```python
from build123d import *

# Parameters (mm, degrees)
F1_DEPTH  = 2
F2_W      = 78
F2_H      = 1.5
F3_DEPTH  = 2
F4_W      = 20
F4_H      = 1.5
F5_DEPTH  = 7
F6_W      = 78
F6_H      = 1.5
F7_DEPTH  = 2
F8_W      = 78
F8_H      = 3
F9_DEPTH  = 3
F10_DEPTH = 2
F11_DEPTH = 2
F12_W     = 3
F12_H     = 11
F13_DEPTH = 5
F14_R     = 5


with BuildPart() as f1:
    # F0 (on Top) → F1 (new body)
    with BuildSketch(Plane.XY):
        with BuildLine():
            Line((7.8453938663, 18.7269745824), (-14.6546061337, 18.7269745824))
            add(Edge.make_bspline(
                [(-14.6546061337, 18.7269745824), (-14.6546061337, 12.4846497216), (-14.9176308165, 6.2423248608), (-15.345167051, 0)],
                knots=[0.5, 0.5, 0.5, 0.5, 0.6872697458, 0.6872697458, 0.6872697458, 0.6872697458], degree=3))
            Line((-15.345167051, 0), (8.5359547836, 0))
            add(Edge.make_bspline(
                [(7.8453938663, 18.7269745824), (7.8453938663, 12.4846497216), (8.1084185491, 6.2423248608), (8.5359547836, 0)],
                knots=[0.5, 0.5, 0.5, 0.5, 0.6872697458, 0.6872697458, 0.6872697458, 0.6872697458], degree=3))
        make_face()
        Polygon((11.5953938663, -31.2730254176), (-18.4046061337, -31.2730254176), (-42.4046061337, -31.2730254176), (-42.4046061337, -34.2730254176), (35.5953938663, -34.2730254176), (35.5953938663, -31.2730254176), align=None)
        with BuildLine():
            Line((8.5359547836, 0), (-15.345167051, 0))
            add(Edge.make_bspline(
                [(-15.345167051, 0), (-16.0591292274, -10.4243418059), (-17.2318676805, -20.8486836117), (-18.4046061337, -31.2730254176)],
                knots=[0.6872697458, 0.6872697458, 0.6872697458, 0.6872697458, 1, 1, 1, 1], degree=3))
            Line((-18.4046061337, -31.2730254176), (11.5953938663, -31.2730254176))
            add(Edge.make_bspline(
                [(8.5359547836, 0), (9.24991696, -10.4243418059), (10.4226554131, -20.8486836117), (11.5953938663, -31.2730254176)],
                knots=[0.6872697458, 0.6872697458, 0.6872697458, 0.6872697458, 1, 1, 1, 1], degree=3))
        make_face()
    extrude(amount=F1_DEPTH)

    # F2 (on face) → F3 (join)
    with BuildSketch(Plane.XY.offset(2)):
        with Locations((-3.4046061337, -33.5230254176)):
            Rectangle(F2_W, F2_H)
    extrude(amount=F3_DEPTH)

    # F4 (on face) → F5 (join)
    with BuildSketch(Plane.XY.offset(4)):
        with Locations((-32.4046061337, -33.5230254176)):
            Rectangle(F4_W, F4_H)
        with Locations((25.5953938663, -33.5230254176)):
            Rectangle(F4_W, F4_H)
    extrude(amount=F5_DEPTH)

    # F6 (on face) → F7 (join)
    with BuildSketch(Plane.XY.offset(11)):
        with Locations((-3.4046061337, -33.5230254176)):
            Rectangle(F6_W, F6_H)
    extrude(amount=F7_DEPTH)

    # F8 (on face) → F9 (join)
    with BuildSketch(Plane.XY.offset(13)):
        with Locations((-3.4046061337, -32.7730254176)):
            Rectangle(F8_W, F8_H)
    extrude(amount=F9_DEPTH)

    # F10 (add): a face of the model
    f10_faces = [f1.faces().sort_by_distance(p)[0] for p in [
        (-3.4046061337, -31.2730254176, 14.5),
    ]]
    extrude(f10_faces, amount=F10_DEPTH)

    # F11 (add): faces of the model
    f11_faces = [f1.faces().sort_by_distance(p)[0] for p in [
        (23.5953938663, -31.2730254176, 1),
        (-30.4046061337, -31.2730254176, 1),
    ]]
    extrude(f11_faces, amount=F11_DEPTH)

    # F12 (on face) → F13 (join)
    with BuildSketch(Plane(origin=(0, -32.7730254176, 0), x_dir=(-1, 0, 0), z_dir=(0, 1, 0))):
        with Locations((40.9046061337, 7.5)):
            Rectangle(F12_W, F12_H)
        with Locations((-34.0953938663, 7.5)):
            Rectangle(F12_W, F12_H)
    extrude(amount=F13_DEPTH)

    # F14
    f14_edges = [f1.edges().sort_by_distance(p)[0] for p in [
        (35.595394, -31.773025, 16),
        (35.595394, -31.773025, 0),
        (-42.404606, -31.773025, 0),
        (-42.404606, -31.773025, 16),
    ]]
    fillet(f14_edges, radius=F14_R)


solid = f1.part
```
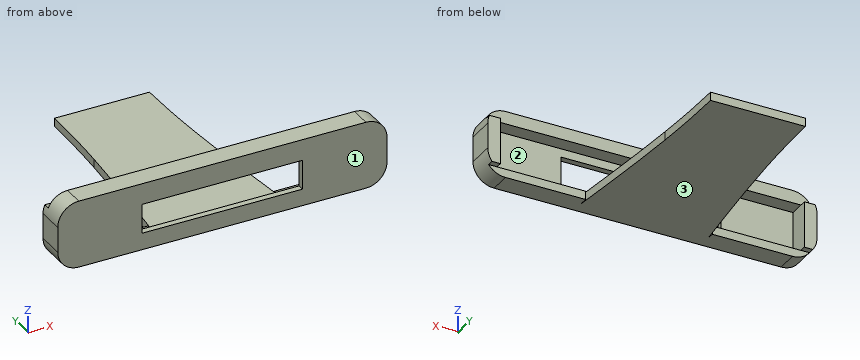
Work out the finished part from the listing and answer in its coordinate system (mm). Face numbers are marked on the shaded views. Round coordinates to 2 decimals unless told otherwise and drop trailing zeros. Order: outer loops, then holes, each group sorted by start corner. A loop starts at its lowest first (then second) coordinate and runs counter-clockwise, first axis right, second up.
Q1. A cutting plane is placed at B-B, the plane x = 1.5. Determine the outline of the cut face in (y, z).
Solution:
outline: (-34.27, 0) - (18.73, 0) - (18.73, 2) - (-32.77, 2) - (-32.77, 4) - (-34.27, 4) - close; (-34.27, 11) - (-32.77, 11) - (-32.77, 13) - (-29.27, 13) - (-29.27, 16) - (-34.27, 16) - close
Q2. The mould has two halves that part along Z. Classify the marked faces 1, 2 and 3: pulls with the +Z half, pulls with the -Z half, needs draft (parallel to the pull), parting line crosses it, or undercut.
Solution:
face 1: needs draft
face 2: undercut
face 3: pulls with the -Z half
Q3. Find the intervals of material crossed by line 1 along Z through (x, y) = (25, -31); line 2 along Y through (x, z) = (-23.5, 1.25); line 3 along Y through (x, z) = (-38, 9), in increasing order.
Solution:
line 1: z = 0 to 2, 13 to 16
line 2: y = -34.27 to -29.27
line 3: y = -34.27 to -32.77
Q4. Given pin 1 Ø1.5 at (x, z) = (-41.5, 8.5) entering from +Y; pin 2 Ø2 at (x, z) = (20, 0.5) entering from +Y; pin 3 Ø1.6 at (y, z) = (-30, 1) entering from +X; pin 4 Ø1.5 at (y, z) = (-26.5, 3.5) entering from +X (3 decimals), each flat-ended and moving along its own axis, determine where each tip first touches the part or whether it passes through.
Solution:
pin 1: stops at y = -27.77
pin 2: stops at y = -29.27
pin 3: stops at x = 34.44
pin 4: passes through
Q5. A cutting plane is placed at A-A, the plane z = 7.75. Determine the outline of the cut face in (x, y).
Solution:
outline: (-42.4, -34.27) - (-22.4, -34.27) - (-22.4, -32.77) - (-39.4, -32.77) - (-39.4, -27.77) - (-42.4, -27.77) - close; (15.6, -34.27) - (35.6, -34.27) - (35.6, -27.77) - (32.6, -27.77) - (32.6, -32.77) - (15.6, -32.77) - close
Q6. A cutting plane is placed at C-C, the plane x = 21.5. Determine the outline of the cut face in (y, z), then the cut area to 3 significant figures.
Solution:
outline: (-34.27, 0) - (-29.27, 0) - (-29.27, 2) - (-32.77, 2) - (-32.77, 13) - (-29.27, 13) - (-29.27, 16) - (-34.27, 16) - close
area: 41.5 mm2
Q7. A cutting plane is placed at D-D, the plane z = 3. Determine the outline of the cut face in (x, y), then the cut area to 3 significant figures.
Solution:
outline: (-41.99, -34.27) - (35.18, -34.27) - (35.18, -27.77) - (32.6, -27.77) - (32.6, -32.77) - (-39.4, -32.77) - (-39.4, -27.77) - (-41.99, -27.77) - close
area: 142 mm2
